from build123d import *

# Parameters (mm, degrees)
F0_R     = 50.8
F0_R_2   = 44.45
F1_DEPTH = 914.4
F2_SIZE  = 5.08
F3_SIZE  = 5.08


with BuildPart() as f1:
    # F0 (on Top) → F1 (new body)
    with BuildSketch(Plane.XY):
        Circle(F0_R)
        Circle(F0_R_2, mode=Mode.SUBTRACT)
    extrude(amount=-F1_DEPTH)

    # F2
    f2_edges = [f1.edges().sort_by_distance(p)[0] for p in [
        (-50.8, 0, 0),
    ]]
    chamfer(f2_edges, length=F2_SIZE)

    # F3
    f3_edges = [f1.edges().sort_by_distance(p)[0] for p in [
        (-50.8, 0, -914.4),
    ]]
    chamfer(f3_edges, length=F3_SIZE)


solid = f1.part
Build history of the part. All positions in model axes, mm. Give positions to 0.01 mm unless a question says otherwise; leave off trailing zeros. Loops run counter-clockwise (first coordinate to the right, second up) from the corner with the lowest first, then second, coordinate; pieces in that order, holes last. Notation, with made-up numbers: (58.5, -9) -> (88.5, -9) arc R22 ccw to (88.5, 2) -> close; hole circle Ø3 at (75.5, 37). An arc over 180 degrees is marked (long way). Answer in a Markdown table with one row per item.
Item 1: Probe line 1 along Y through (x, z) = (0, -523); line 2 along X through (y, z) = (3, -541); line 3 along Y through (x, z) = (-35.5, -573). List the from-to ranges inside material, lowest first. Write a range as [from, to].
Findings below:
| item | result |
|---|---|
| line 1 | y = [-50.8, -44.45], [44.45, 50.8] |
| line 2 | x = [-50.71, -44.35], [44.35, 50.71] |
| line 3 | y = [-36.34, -26.75], [26.75, 36.34] |
Item 2: Mould opens along Y. For faces 1 (the flat face through (-7, 44.2, 0)), 2 (the cylindrical face through (-11.012, -49.592, -450.87)), 3 (the cylindrical face through (42.397, 13.352, -450.799)) say: pulls with the +Y half, pulls with the -Y half, needs draft (parallel to the pull), parting line crosses it, or undercut.
Findings below:
| item | result |
|---|---|
| face 1 | needs draft |
| face 2 | parting line crosses it |
| face 3 | undercut |
Item 3: Flat gauge pins, fed straight in: P1, Ø5, axis at y = 28, z = -818, coming from the -X side; P2, Ø2, axis at x = 38, z = -330, coming from the +Y side; P3, Ø6, axis at x = 5, z = -271.5, coming from the +Y side. Where does each tip first touch, or does it go through?
Findings below:
| item | result |
|---|---|
| P1 | stops at x = -43.94 |
| P2 | stops at y = 34.81 |
| P3 | stops at y = 50.76 |
Item 4: Slice it at A-A on x = 0. Write the cut outline in (y, z), plus the area to 3 significant figures.
Findings below:
| item | result |
|---|---|
| outline | (-50.8, -909.32) -> (-45.72, -914.4) -> (-44.45, -914.4) -> (-44.45, 0) -> (-45.72, 0) -> (-50.8, -5.08) -> close; (44.45, -914.4) -> (45.72, -914.4) -> (50.8, -909.32) -> (50.8, -5.08) -> (45.72, 0) -> (44.45, 0) -> close |
| area | 11,600 mm² |
Item 5: Slice it at C-C on z = -718. Write the cut outline in (x, y), plus the area to 3 significant figures.
Findings below:
| item | result |
|---|---|
| outline | circle Ø101.6 at (0, 0); hole circle Ø88.9 at (0, 0) |
| area | 1,900 mm² |
